Autodesk Inventor part; units mm, degrees
ref_plane "YZ Plane" through (0, 0, 0) normal (1, 0, 0) x (0, 1, 0)
ref_plane "XZ Plane" through (0, 0, 0) normal (0, 1, 0) x (-1, 0, 0)
ref_plane "XY Plane" through (0, 0, 0) normal (0, 0, 1) x (1, 0, 0)
sketch "スケッチ1" plane through (0, 0, 0) normal (1, 0, 0) x (0, 1, 0)
  circle A0 centre (0, 0) radius 10
  circle A1 centre (0, -10) radius 1.35
  circle A2 centre (8.6603, 5) radius 1.35
  circle A3 centre (-8.6603, 5) radius 1.35
  circle A4 centre (0, 0) radius 5
  line L0 (0, 0) -> (0, 50)
  circle A5 centre (0, 50) radius 22.5
  circle A6 centre (0, 0) radius 14
  line L1 (-14, 0) -> (-22.5, 50)
  line L2 (14, 0) -> (22.5, 50)
  line L3 (0, -14) -> (-11.62, -14)
  line L4 (-11.62, -14) -> (-14, 0)
  line L5 (0, -14) -> (11.62, -14)
  line L6 (11.62, -14) -> (14, 0)
  line L7 (0, 20) -> (-17.4, 20)
  line L8 (0, 20) -> (17.4, 20)
  dimension "d0" = 20
  dimension "d1" = 2.7
  dimension "d4" = 360
  dimension "d6" = 10
  dimension "d7" = 50
  dimension "d8" = 45
  dimension "d9" = 28
extrude "押し出し1" add sketch "スケッチ1" along normal blind 4 contours A0 A1 A3 A2 | A6 L6 L4 | A6 L1 L7 L0 | L0 L8 L2 A6 | L6 L5 A6 | A6 L3 L4
sketch "スケッチ2" plane through (0, -17.4, 20) normal (0, 0, 1) x (1, 0, 0)
  line L0 (0, 17.4) -> (30, 17.4)
  circle A0 centre (30, 17.4) radius 22.5
  circle A1 centre (30, 17.4) radius 18.5
  circle A2 centre (30, 17.4) radius 14.25
  circle A3 centre (48.5, 17.4) radius 1.35
  circle A4 centre (20.75, 33.4215) radius 1.35
  circle A5 centre (20.75, 1.3785) radius 1.35
  line L1 (0, 29.02) -> (0, 34.8)
  line L2 (0, 0) -> (0, 5.78)
  line L3 (0, 34.8) -> (0, 0)
  line L4 (4, 29.02) -> (4, 34.8)
  line L5 (4, 34.8) -> (7, 34.8)
  line L6 (7, 34.8) -> (30, 39.9)
  line L7 (4, 0) -> (4, 5.78)
  line L8 (4, 0) -> (7, 0)
  line L9 (7, 0) -> (30, -5.1)
  line L10 (4, 0) -> (0, 0)
  line L11 (0, 34.8) -> (4, 34.8)
  line L12 (0, 0) -> (0, 34.8)
  line L13 (0, 34.8) -> (4, 34.8)
  dimension "d14" = 37
  dimension "d12" = 30
  dimension "d13" = 45
  dimension "d15" = 28.5
  dimension "d16" = 2.7
  dimension "d19" = 360
  dimension "d21" = 3
  dimension "d22" = 3
extrude "押し出し2" add sketch "スケッチ2" along normal blind 4 contours L3 L1 L11 L5 L6 A0 L0 | L0 A0 L9 L8 L10 L2 L3 | A1 A4 A3 A5 | A0 L6 L9
fillet "フィレット1" radius 3 2 edges at (4, 0, 20) (0, 0, 24)
fillet "フィレット2" radius 3 2 edges at (2, -11.62, -14) (2, 11.62, -14)
sketch "スケッチ7" plane through (0, -17.4, 24) normal (0, 0, 1) x (1, 0, 0)
  circle A0 centre (30, 17.4) radius 14.25
  line L0 (30, 17.4) -> (182.95, 17.4)
  line L1 (30, 17.4) -> (182.95, 17.4) construction
  circle A1 centre (182.95, 17.4) radius 3.5
  circle A2 centre (182.95, 17.4) radius 10
  line L2 (182.95, 27.4) -> (50.1556, 27.4)
  arc A3 (30, -5.1) -> (30, 39.9) centre (30, 17.4) ccw
  line L3 (182.95, 27.4) -> (315.7444, 27.4) construction
  line L4 (182.95, 7.4) -> (50.1556, 7.4)
  point P0 (0, 17.4)
  dimension "d55" = 152.95
  dimension "d56" = 0
  dimension "d57" = 7
  dimension "d58" = 20
  dimension "d59" = 180
extrude "押し出し7" add sketch "スケッチ7" against normal blind 4 contours A3 L2 A2 L0 | L0 A2 L4 A3 | A2
sketch "スケッチ8" plane through (0, -17.4, 24) normal (0, 0, 1) x (1, 0, 0)
  circle A0 centre (20.75, 33.4215) radius 1.35
  circle A1 centre (20.75, 33.4215) radius 2.5
  circle A2 centre (48.5, 17.4) radius 1.35
  circle A3 centre (48.5, 17.4) radius 2.5
  circle A4 centre (20.75, 1.3785) radius 1.35
  circle A5 centre (20.75, 1.3785) radius 2.5
  point P0 (0, 17.4)
  dimension "d63" = 5
  dimension "d64" = 5
  dimension "d65" = 5
extrude "押し出し8" cut sketch "スケッチ8" against normal blind 2 contours A0 | A1 | A3 | A4 | A5
fillet "フィレット4" radius 2 1 edges at (50.1556, 10, 22)
sketch "スケッチ12" plane through (0, -17.4, 24) normal (0, 0, 1) x (1, 0, 0)
  circle A0 centre (48.5, 17.4) radius 2.5
  circle A1 centre (20.75, 1.3785) radius 2.5
  circle A2 centre (20.75, 33.4215) radius 2.5
  circle A3 centre (182.95, 17.4) radius 3.5
  line L0 (3, 0) -> (3, 34.8)
  line L1 (3, 0) -> (7, 0)
  line L2 (7, 0) -> (30, -5.1)
  arc A4 (30, -5.1) -> (50.1556, 7.4) centre (30, 17.4) ccw
  line L3 (50.1556, 7.4) -> (182.95, 7.4)
  arc A5 (182.95, 7.4) -> (182.95, 27.4) centre (182.95, 17.4) ccw
  line L4 (182.95, 27.4) -> (51.36, 27.4)
  arc A6 (49.6163, 28.4204) -> (51.36, 27.4) centre (51.36, 29.4) ccw
  arc A7 (49.6163, 28.4204) -> (30, 39.9) centre (30, 17.4) ccw
  line L5 (30, 39.9) -> (7, 34.8)
  line L6 (7, 34.8) -> (3, 34.8)
  circle A8 centre (30, 17.4) radius 14.25
  line L7 (182.95, 7.4) -> (232.95, 7.4)
  line L8 (182.95, 27.4) -> (232.95, 27.4)
  line L9 (232.95, 27.4) -> (232.95, 7.4)
  point P0 (0, 17.4)
  dimension "d92" = 50
  dimension "d93" = 50
extrude "押し出し12" add sketch "スケッチ12" against normal blind 4 contours A5 L8 L9 L7
sketch "スケッチ13" plane through (0, -17.4, 24) normal (0, 0, 1) x (1, 0, 0)
  circle A0 centre (48.5, 17.4) radius 2.5
  circle A1 centre (20.75, 1.3785) radius 2.5
  circle A2 centre (20.75, 33.4215) radius 2.5
  circle A3 centre (182.95, 17.4) radius 3.5
  line L0 (3, 0) -> (3, 34.8)
  line L1 (3, 0) -> (7, 0)
  line L2 (7, 0) -> (30, -5.1)
  arc A4 (30, -5.1) -> (50.1556, 7.4) centre (30, 17.4) ccw
  line L3 (50.1556, 7.4) -> (232.95, 7.4)
  line L4 (232.95, 7.4) -> (232.95, 27.4)
  line L5 (232.95, 27.4) -> (51.36, 27.4)
  arc A5 (49.6163, 28.4204) -> (51.36, 27.4) centre (51.36, 29.4) ccw
  arc A6 (49.6163, 28.4204) -> (30, 39.9) centre (30, 17.4) ccw
  line L6 (30, 39.9) -> (7, 34.8)
  line L7 (7, 34.8) -> (3, 34.8)
  circle A7 centre (30, 17.4) radius 14.25
  line L8 (197.95, 24.9) -> (182.95, 27.4)
  line L9 (197.95, 9.9) -> (182.95, 7.4)
  line L10 (197.95, 9.9) -> (228.95, 9.9)
  line L11 (228.95, 9.9) -> (228.95, 24.9)
  line L12 (228.95, 24.9) -> (197.95, 24.9)
  point P0 (0, 17.4)
  dimension "d96" = 2.5
  dimension "d97" = 15
  dimension "d98" = 35
  dimension "d99" = 35
  dimension "d100" = 31
  dimension "d101" = 15
  dimension "d102" = 31
extrude "押し出し13" cut sketch "スケッチ13" against normal blind 4 contours L9 L10 L11 L12 L8 L5 L4 L3
sketch "スケッチ14" plane through (0, -17.4, 24) normal (0, 0, 1) x (1, 0, 0)
  circle A0 centre (30, 17.4) radius 14.25
  line L0 (182.95, 7.4) -> (197.95, 9.9)
  line L1 (197.95, 9.9) -> (228.95, 9.9)
  line L2 (228.95, 9.9) -> (228.95, 24.9)
  line L3 (228.95, 24.9) -> (197.95, 24.9)
  line L4 (197.95, 24.9) -> (182.95, 27.4)
  line L5 (182.95, 27.4) -> (51.36, 27.4)
  arc A1 (49.6163, 28.4204) -> (51.36, 27.4) centre (51.36, 29.4) ccw
  arc A2 (49.6163, 28.4204) -> (30, 39.9) centre (30, 17.4) ccw
  line L6 (30, 39.9) -> (7, 34.8)
  line L7 (7, 34.8) -> (3, 34.8)
  line L8 (3, 0) -> (3, 34.8)
  line L9 (3, 0) -> (7, 0)
  line L10 (7, 0) -> (30, -5.1)
  arc A3 (30, -5.1) -> (50.1556, 7.4) centre (30, 17.4) ccw
  line L11 (50.1556, 7.4) -> (182.95, 7.4)
  circle A4 centre (182.95, 17.4) radius 3.5
  circle A5 centre (20.75, 33.4215) radius 2.5
  circle A6 centre (20.75, 1.3785) radius 2.5
  circle A7 centre (48.5, 17.4) radius 2.5
  line L12 (197.95, 24.9) -> (197.95, 13.9)
  line L13 (197.95, 13.9) -> (224.95, 13.9)
  line L14 (224.95, 13.9) -> (224.95, 20.9)
  line L15 (224.95, 20.9) -> (217.95, 20.9)
  line L16 (217.95, 20.9) -> (217.95, 24.9)
  point P0 (0, 17.4)
  dimension "d105" = 4
  dimension "d106" = 4
  dimension "d107" = 4
  dimension "d108" = 4
  dimension "d109" = 4
  dimension "d110" = 7
  dimension "d113" = 27
  dimension "d114" = 4
extrude "押し出し14" cut sketch "スケッチ14" against normal blind 4 contours L16 L15 L14 L13 L12 L3
fillet "フィレット7" radius 1 11 edges at (197.95, -7.5, 22) (182.95, -10, 22) (228.95, -7.5, 22) (217.95, 3.5, 22) (224.95, 3.5, 22) (217.95, 7.5, 22) (228.95, 7.5, 22) (182.95, 10, 22) (197.95, 7.5, 22) (197.95, -3.5, 22) (224.95, -3.5, 22)
equation "\"d99\" = d98"
equation "\"d102\" = d100"
equation "\"d106\" = d105"
equation "\"d107\" = d105"
equation "\"d108\" = d105"
equation "\"d109\" = d105"
equation "\"d114\" = d105"
properties part number "motor_holder_8-4" material "ABS プラスチック"
The model under review builds one solid part; all positions refer to its coordinate system, in mm. A direction names the side the tool comes from. Give positions to 0.01 mm unless a question says otherwise; leave off trailing zeros. Write each loop counter-clockwise with the first axis right and the second up, starting at its lowest first coordinate (ties: lowest second). Pieces come first, ordered by that corner, then holes. Notation, with made-up numbers: (-24, 89.25) - (2, 89.25) arc R20 ccw to (2, 95.25) - close; hole circle Ø1 at (-17, -5.5). An arc over 180 degrees is marked (long way). Answer in a Markdown table with one row per item. Add a question column.
1. Tool access review of faces 5 (the flat face through (224, 7.5, 22)), 6 (the flat face through (213, -7.5, 22)), 7 (the flat face through (50, -1, 22)), 8 (the flat face through (221, 3.5, 22)), 9 (the flat face through (3, 17.4, 22)): name each direction out of +Z, -Z, +X, -X, +Y, -Y from which nothing blocks a thin tool from reaching the whole face with its end or side.
2. Wall thickness on line 1 along Y through (x, z) = (20, 21); line 2 along X through (y, z) = (1, 21); line 3 along Z through (x, y) = (197, -4.5): over which ranges is each line inside the solid? List them lowest first. Write a range as [from, to].
3. We need section A-A on x = 68.5. Write out the cut boundary in (y, z), then the cut area to 3 significant figures.
4. Insertion check: P1, Ø2, axis at y = 8.5, z = 7, coming from the +X side; P2, Ø6, axis at x = 20.75, y = 16.02, coming from the -Z side; P3, Ø3, axis at x = 137.5, z = 22.5, coming from the +Y side. Each pin has a flat end and moves straight along its axis. Give the tip position at first contact, or say it passes through.
5. We need section B-B on z = 14.5. Write out the cut boundary in (x, y) (3 decimals), then the cut area to 3 significant figures.
6. Draft analysis for pull direction Y (two halves, no side actions). For faces 1 (the flat face through (197.95, 2, 22)), 2 (the flat face through (18.339, -19.914, 21.972)), 3 (the cylindrical face through (50.81, -0.96, 23.01)), 4 (the cylindrical face through (1.97, -1.08, 4.88)), state which applies: +Y half, -Y half, draft (parallel to the pull), parting line (faces both ways), or undercut.
Ans:
| question | item | result |
|---|---|---|
| 1 | face 5 | +Z, -Z, +X, +Y |
| 1 | face 6 | +Z, -Z, +X, -Y |
| 1 | face 7 | +Z |
| 1 | face 8 | +Z, -Z |
| 1 | face 9 | +Z, -Z, -X, +Y |
| 2 | line 1 | y = [-20.28, -17.14], [-14.9, -10.15], [10.15, 14.9], [17.14, 20.28] |
| 2 | line 2 | x = [0, 15.79], [44.21, 47.59], [49.41, 179.6], [186.3, 197.95], [224.95, 228.95] |
| 2 | line 3 | z = [20, 24] |
| 3 | outline | (-10, 20) - (10, 20) - (10, 24) - (-10, 24) - close |
| 3 | area | 80.0 mm^2 |
| 4 | P1 | stops at x = 4 |
| 4 | P2 | stops at z = 20 |
| 4 | P3 | stops at y = 10 |
| 5 | outline | (0, -16.465) - (4, -16.465) - (4, 16.465) - (0, 16.465) - close |
| 5 | area | 132 mm^2 |
| 6 | face 1 | draft |
| 6 | face 2 | -Y half |
| 6 | face 3 | undercut |
| 6 | face 4 | undercut |
